Work out the finished part from the listing and answer in its coordinate system (mm). A direction names the side the tool comes from. Round coordinates to 2 decimals unless told otherwise and drop trailing zeros.
1. A tool of negligible diameter and unlimited length cuts with its end or side. For faces 4 (the face through (-47.67, 1.76, 5.75)), 5 (the face through (61, -28.57, 3.04)), 6 (the face through (26.686, 30.246, 3.143)), from which of +Z, -Z, +X, -X, +Y, -Y can it reach the whole face along a straight path? Write none if from no direction.
2. Flat-ended cylindrical pins translate along their axes: pin 1 Ø12 at (x, y) = (-33, -6.5) entering from -Z; pin 2 Ø1.5 at (x, z) = (-49, 4) entering from +Y; pin 3 Ø9.5 at (x, y) = (-53.26, 0) entering from +Z. Find the tip coordinate at first contact, or state that the pin passes through.
3. Determine the mould class of faces 1 (the face through (-62.5, 0, 3)), 2 (the face through (30.4, 30.25, 3.53)), 3 (the face through (61.07, 28.5, 3.04)) for opening direction X: pulls with the +X half, pulls with the -X half, needs draft (parallel to the pull), parting line crosses it, or undercut.
4. A straight line is drawn through the part: probe 1 along Y at (x, z) = (-43, 3.4). Find the intervals that lie inside material, in ascending order.
```python
from build123d import *

# Parameters (mm, degrees)
F0_W     = 125
F0_H     = 60
F1_DEPTH = 6
F2_R     = 5
F3_R     = 5
F4_R     = 1.925177
F5_DEPTH = 0.5
F6_R     = 1.925177
F7_DEPTH = 0.5
F8_R     = 5.863053
F9_DEPTH = 0.5


with BuildPart() as f1:
    # F0 (on Top) → F1 (new body)
    with BuildSketch(Plane.XY):
        Rectangle(F0_W, F0_H)
    extrude(amount=F1_DEPTH)

    # F2
    f2_edges = [f1.edges().sort_by_distance(p)[0] for p in [
        (-62.5, 30, 3),
        (62.5, 30, 3),
        (62.5, -30, 3),
    ]]
    fillet(f2_edges, radius=F2_R)

    # F3
    f3_edges = [f1.edges().sort_by_distance(p)[0] for p in [
        (-62.5, -30, 3),
    ]]
    fillet(f3_edges, radius=F3_R)

    # F4 (on face) → F5 (join)
    with BuildSketch(Plane(origin=(0, 30, 0), x_dir=(-1, 0, 0), z_dir=(0, 1, 0))):
        with Locations((-32.237682, 2.95109)):
            Circle(F4_R)
    extrude(amount=F5_DEPTH)

    # F6 (on face) → F7 (join)
    with BuildSketch(Plane(origin=(0, 30, 0), x_dir=(-1, 0, 0), z_dir=(0, 1, 0))):
        with Locations((-24.762407, 3.057879)):
            Circle(F6_R)
    extrude(amount=F7_DEPTH)

    # F8 (on face) → F9 (cut)
    with BuildSketch(Plane.XY.offset(6)):
        with Locations((-53.260919, 0)):
            Circle(F8_R)
    extrude(amount=-F9_DEPTH, mode=Mode.SUBTRACT)


solid = f1.part
```
Worked answers:
1. face 4: +Z
1. face 5: +Z, -Z, +X, -Y
1. face 6: +Y
2. pin 1: stops at z = 0
2. pin 2: stops at y = 30
2. pin 3: stops at z = 5.5
3. face 1: pulls with the -X half
3. face 2: undercut
3. face 3: pulls with the +X half
4. probe 1: y = -30 to 30
